Design review of the part built by this model. Coordinates are the model's own, in mm. Coordinates: 2 decimals unless noted, no trailing zeros. Loops run counter-clockwise (first coordinate to the right, second up) from the corner with the lowest first, then second, coordinate; pieces in that order, holes last. Notation, with made-up numbers: M -1.5,32.25 L 8.5,32.25 A27 cw 8.5,56.25 Z; hole C -3.5,20 d1. An arc over 180 degrees is marked long. Answer as a JSON object with one key per item and string values. Group by question number.
1. To check wall thickness, follow probe 1 along Z at (x, y) = (0.5, 371); probe 2 along Y at (x, z) = (-74.5, 33); probe 3 along Z at (x, y) = (27.5, 304.5). State the ranges of each line that lie inside material, in increasing order.
2. Consider section C-C (y = 51). State the section outline as (x, z) points, then the cut area to 3 significant figures.
3. Insertion check: pin 1 (10 mm diameter, centred on x = 92, z = 59, fed in from +Y); pin 2 (10 mm diameter, centred on y = 234.5, z = 31.5, fed in from -X); pin 3 (10 mm diameter, centred on y = 209, z = 32, fed in from -X). Each pin has a flat end and moves straight along its axis. Give the tip position at first contact, or say it passes through.
4. Draft analysis for pull direction Y (two halves, no side actions). For faces 1 (the flat face through (-1, 450.85, 1)), 2 (the cylindrical face through (35.069, 224.804, -67.425)), 3 (the conical face through (-15.444, 0.243, -69.549)), 4 (the flat face through (-2, -25, 2)), state which applies: +Y half, -Y half, draft (parallel to the pull), parting line (faces both ways), or undercut.
5. Consider section B-B (x = 0). State the section outline as (y, z) points, then the cut area to 3 significant figures.
6. Consider section D-D (x = -100). State the section outline as (y, z) points, then the cut area to 3 significant figures.
7. Consider section A-A (z = 0). State the section outline as (x, y) points.
from build123d import *

# Parameters (mm, degrees)
F0_R     = 76
F1_DEPTH = 450.85
F2_SIZE  = 5
F3_R     = 135.146802
F4_DEPTH = 25


with BuildPart() as f1:
    # F0 (on Front) → F1 (new body)
    with BuildSketch(Plane.XZ):
        Circle(F0_R)
    extrude(amount=-F1_DEPTH)

    # F2
    f2_edges = [f1.edges().sort_by_distance(p)[0] for p in [
        (-76, 0, 0),
    ]]
    chamfer(f2_edges, length=F2_SIZE)

    # F3 (on Front) → F4 (join)
    with BuildSketch(Plane.XZ):
        Circle(F3_R)
    extrude(amount=F4_DEPTH)


solid = f1.part
Findings below:
{
 "1": {"probe 1": "z = -76 to 76", "probe 2": "y = -25 to 0", "probe 3": "z = -70.85 to 70.85"},
 "2": {"outline": "C 0,0 d152", "area": "18,100 mm^2"},
 "3": {"pin 1": "stops at y = 0", "pin 2": "stops at x = -71.23", "pin 3": "stops at x = -71.04"},
 "4": {"face 1": "+Y half", "face 2": "draft", "face 3": "undercut", "face 4": "-Y half"},
 "5": {"outline": "M -25,-135.15 L 0,-135.15 L 0,-71 L 5,-76 L 450.85,-76 L 450.85,76 L 5,76 L 0,71 L 0,135.15 L -25,135.15 Z", "area": "75,300 mm^2"},
 "6": {"outline": "M -25,-90.91 L 0,-90.91 L 0,90.91 L -25,90.91 Z", "area": "4,550 mm^2"},
 "7": {"outline": "M -135.15,-25 L 135.15,-25 L 135.15,0 L 71,0 L 76,5 L 76,450.85 L -76,450.85 L -76,5 L -71,0 L -135.15,0 Z"}
}
